```python
from build123d import *

# Parameters (mm, degrees)
F0_W     = 5
F0_H     = 2.5
F1_DEPTH = 18.7
F2_DEPTH = 36.3
F3_R     = 1.75
F4_DEPTH = 15.001


with BuildPart() as f1:
    # F0 (on Top) → F1 (new body, symmetric)
    with BuildSketch(Plane.XY):
        with Locations((2.5, 1.25)):
            Rectangle(F0_W, F0_H)
        with Locations((-2.5, 1.25)):
            Rectangle(F0_W, F0_H)
    extrude(amount=F1_DEPTH, both=True)

    # F0 (on Top) → F2 (join, symmetric)
    with BuildSketch(Plane.XY):
        Polygon((5, 7.6), (5, 2.5), (5, 0), (7.5, 0), (7.5, 7.6), align=None)
        Polygon((-5, 7.6), (-7.5, 7.6), (-7.5, 0), (-5, 0), (-5, 2.5), align=None)
    extrude(amount=F2_DEPTH, both=True)

    # F3 (on face) → F4 (cut, through all)
    with BuildSketch(Plane.YZ.offset(7.5)):
        with Locations((3.8, 32.5)):
            Circle(F3_R)
        Polygon((0, 36.3), (3.8, 36.3), (7.6, 36.3), (7.6, 42.815186), (0, 42.815186), align=None)
        with BuildLine():
            ThreePointArc((3.8, 36.3), (6.487006, 35.187006), (7.6, 32.5))
            Line((7.6, 32.5), (7.6, 36.3))
            Line((7.6, 36.3), (3.8, 36.3))
        make_face()
        with BuildLine():
            Line((0, 36.3), (0, 32.5))
            ThreePointArc((0, 32.5), (1.112994, 35.187006), (3.8, 36.3))
            Line((3.8, 36.3), (0, 36.3))
        make_face()
        with Locations((3.8, -32.5)):
            Circle(F3_R)
        Polygon((7.6, -36.3), (3.8, -36.3), (0, -36.3), (0, -42.815186), (7.6, -42.815186), align=None)
        with BuildLine():
            Line((7.6, -36.3), (7.6, -32.5))
            ThreePointArc((7.6, -32.5), (6.487006, -35.187006), (3.8, -36.3))
            Line((3.8, -36.3), (7.6, -36.3))
        make_face()
        with BuildLine():
            ThreePointArc((3.8, -36.3), (1.112994, -35.187006), (0, -32.5))
            Line((0, -32.5), (0, -36.3))
            Line((0, -36.3), (3.8, -36.3))
        make_face()
    extrude(amount=-F4_DEPTH, mode=Mode.SUBTRACT)


solid = f1.part
```
Can you work these out from the model? Positions are in its coordinate system, mm. A direction names the side the tool comes from. Round coordinates to 2 decimals unless told otherwise and drop trailing zeros. Loops run counter-clockwise (first coordinate to the right, second up) from the corner with the lowest first, then second, coordinate; pieces in that order, holes last. Notation, with made-up numbers: (-5, 61.5) -> (2, 61.5) arc R13 ccw to (2, 84.5) -> close; hole circle Ø1 at (40, 46). An arc over 180 degrees is marked (long way). One line per item, written item: value. Start each with the question number.
1. If we section it at B-B, the plane y = 6.5: Write out the boundary of the cut face in (x, z).
2. If I drill on probe 1 along Z at (x, y) = (6.4, 3.8); probe 2 along X at (y, z) = (2.75, 8.5); probe 3 along Y at (x, z) = (-2, 14), over which ranges is the centre line in solid material (lowest first)?
3. For faces 1 (the flat face through (0, 2.5, 0)), 2 (the flat face through (0, 1, 18.7)), 3 (the cylindrical face through (6.3, 4.7, 34)), which set-ups out of +Z, -Z, +X, -X, +Y, -Y let a thin tool reach every point of the face, with its end or its side?
4. If we section it at C-C, the plane z = 7: Write out the boundary of the cut face in (x, y).
5. If we section it at A-A, the plane z = -23.5: Write out the boundary of the cut face in (x, y).
6. For pin 1 (3 mm diameter, centred on x = 0, y = 0.5, fed in from -Z); pin 2 (4 mm diameter, centred on x = 1, y = 2.5, fed in from +Z); pin 3 (5 mm diameter, centred on x = 0, z = -3.5, fed in from +Y), each with a flat end and sliding along its axis, tell me the tip position at first contact or that it passes through.
7. If we mould it in two halves opening along Z, with no side actions, what happens to faces 4 (the flat face through (0, 0, 0)), 5 (the flat face through (0, 1, -18.7)), 6 (the cylindrical face through (-6.232, 5.417, -33.17))? For each: pulls with the +Z half, pulls with the -Z half, needs draft (parallel to the pull), parting line crosses it, or undercut.
8. If we section it at D-D, the plane x = -2.5: Write out the boundary of the cut face in (y, z).
Calculated:
1. outline: (-7.5, -35.17) -> (-5, -35.17) -> (-5, 35.17) -> (-7.5, 35.17) -> close; (5, -35.17) -> (7.5, -35.17) -> (7.5, 35.17) -> (5, 35.17) -> close
2. probe 1: z = -36.3 to -34.25, -30.75 to 30.75, 34.25 to 36.3
2. probe 2: x = -7.5 to -5, 5 to 7.5
2. probe 3: y = 0 to 2.5
3. face 1: +Z, -Z, +Y
3. face 2: +Z, +Y, -Y
3. face 3: +X, -X
4. outline: (-7.5, 0) -> (7.5, 0) -> (7.5, 7.6) -> (5, 7.6) -> (5, 2.5) -> (-5, 2.5) -> (-5, 7.6) -> (-7.5, 7.6) -> close
5. outline: (-7.5, 0) -> (-5, 0) -> (-5, 7.6) -> (-7.5, 7.6) -> close; (5, 0) -> (7.5, 0) -> (7.5, 7.6) -> (5, 7.6) -> close
6. pin 1: stops at z = -18.7
6. pin 2: stops at z = 18.7
6. pin 3: stops at y = 2.5
7. face 4: needs draft
7. face 5: pulls with the -Z half
7. face 6: undercut
8. outline: (0, -18.7) -> (2.5, -18.7) -> (2.5, 18.7) -> (0, 18.7) -> close
